Here's how the part is built. I have some questions about the finished solid (model axes, mm). Coordinates: 2 decimals unless noted, no trailing zeros. Write each loop counter-clockwise with the first axis right and the second up, starting at its lowest first coordinate (ties: lowest second). Pieces come first, ordered by that corner, then holes.
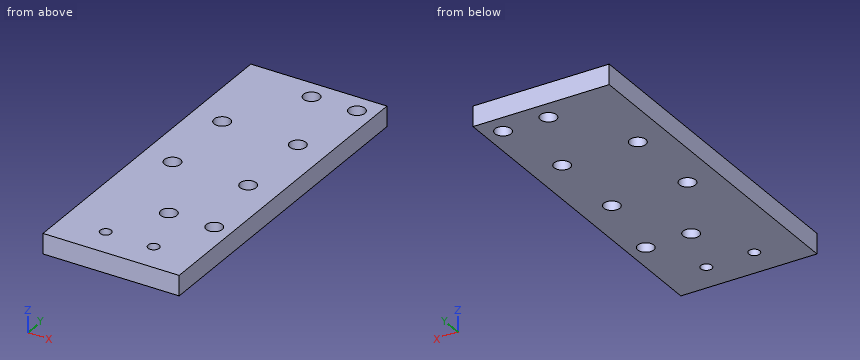
Autodesk Inventor part; units mm, degrees
ref_plane "YZ Plane" through (0, 0, 0) normal (1, 0, 0) x (0, 1, 0)
ref_plane "XZ Plane" through (0, 0, 0) normal (0, 1, 0) x (-1, 0, 0)
ref_plane "XY Plane" through (0, 0, 0) normal (0, 0, 1) x (1, 0, 0)
sketch "Эскиз1" plane through (0, 0, 0) normal (0, 0, 1) x (1, 0, 0)
  circle A0 centre (-7.5, -6.95) radius 1.5 construction
  circle A1 centre (7.5, -6.95) radius 1.5 construction
  circle A2 centre (7.5, -22.95) radius 1.5 construction
  circle A3 centre (-7.5, -22.95) radius 1.5 construction
  circle A4 centre (-7.5, -6.95) radius 1.6
  circle A5 centre (7.5, -6.95) radius 1.6
  circle A6 centre (7.5, -22.95) radius 1.6
  circle A7 centre (-7.5, -22.95) radius 1.6
  line L0 (9, 4.1) -> (-9, 4.1) construction
  line L1 (9, -34) -> (-9, -34) construction
  line L2 (-13.5, 12.05) -> (13.5, 12.05)
  line L3 (13.5, 12.05) -> (13.5, -41.95)
  line L4 (13.5, -41.95) -> (-13.5, -41.95)
  line L5 (-13.5, -41.95) -> (-13.5, 12.05)
  line L6 (-7.5, -6.95) -> (-7.5, 12.05) construction
  line L7 (-7.5, -22.95) -> (-7.5, -41.95) construction
  point P0 (0, 0)
  dimension "d0" = 3.2
  dimension "d1" = 3.2
  dimension "d2" = 3.2
  dimension "d3" = 3.2
  dimension "d4" = 6
  dimension "d5" = 6
  dimension "d8" = 54
extrude "Выдавливание1" add sketch "Эскиз1" along normal blind 4
sketch "Эскиз3" plane through (0, 0, 4) normal (0, 0, 1) x (1, 0, 0)
  circle A0 centre (1, -37.95) radius 2.1 construction
  circle A1 centre (10, -37.95) radius 2.1 construction
  circle A2 centre (1, 8.05) radius 2.1 construction
  circle A3 centre (10, 8.05) radius 2.1 construction
  circle A4 centre (1, -37.95) radius 1.6
  circle A5 centre (10, -37.95) radius 1.6
  circle A6 centre (1, 8.05) radius 1.6
  circle A7 centre (10, 8.05) radius 1.6
  point P0 (0, 0)
  dimension "d9" = 3.2
  dimension "d10" = 3.2
  dimension "d11" = 3.2
  dimension "d12" = 3.2
extrude "Выдавливание2" cut sketch "Эскиз3" against normal blind 10
sketch "Эскиз4" plane through (-13.5, -41.95, 0) normal (0, -1, 0) x (1, 0, 0)
  line L0 (0, 4) -> (27, 4)
  line L1 (0, 0) -> (0, 4)
  line L2 (0, 0) -> (27, 0)
  line L3 (27, 0) -> (27, 4)
  point P0 (13.5, 0)
extrude "Выдавливание3" add sketch "Эскиз4" along normal blind 13
sketch "Эскиз5" plane through (0, 0, 4) normal (0, 0, 1) x (1, 0, 0)
  circle A0 centre (-4.75, -48.95) radius 1.1
  circle A1 centre (4.75, -48.95) radius 1.1
  line L0 (13.5, -54.95) -> (-13.5, -54.95)
  line L1 (-4.75, -48.95) -> (4.75, -48.95) construction
  line L2 (-13.5, -54.95) -> (13.5, -54.95)
  line L3 (0, -54.95) -> (0, -44.9409) construction
  point P0 (0, 0)
  point P1 (0, -48.95)
  dimension "d17" = 2.2
  dimension "d18" = 2.2
  dimension "d19" = 6
  dimension "d20" = 6
  dimension "d21" = 9.5
extrude "Выдавливание4" cut sketch "Эскиз5" against normal blind 13
properties part number "фанера_каретка" material "Древесина (береза)"
1) I need wall thicknesses on probe 1 along Y at (x, z) = (10, 2.15); probe 2 along Y at (x, z) = (-7.5, 3.15); probe 3 along Y at (x, z) = (-4.75, 1.55). Which ranges of each line are inside material? Lowest first, please.
Values follow:
probe 1: y = -54.95 to -39.55, -36.35 to 6.45, 9.65 to 12.05
probe 2: y = -54.95 to -24.55, -21.35 to -8.55, -5.35 to 12.05
probe 3: y = -54.95 to -50.05, -47.85 to 12.05
2) Imagine slicing it at D-D on x = -4.75. Please give me the cut outline in (y, z), then the cut area to 3 significant figures.
Values follow:
outline: (-54.95, 0) - (-50.05, 0) - (-50.05, 4) - (-54.95, 4) - close; (-47.85, 0) - (12.05, 0) - (12.05, 4) - (-47.85, 4) - close
area: 259 mm2
3) Imagine slicing it at B-B on y = -22.95. Please give me the cut outline in (x, z), then the cut area to 3 significant figures.
Values follow:
outline: (-13.5, 0) - (-9.1, 0) - (-9.1, 4) - (-13.5, 4) - close; (-5.9, 0) - (5.9, 0) - (5.9, 4) - (-5.9, 4) - close; (9.1, 0) - (13.5, 0) - (13.5, 4) - (9.1, 4) - close
area: 82.4 mm2
4) Will this pin go through, and if not, where does the flat tip stop? pin 1 (2.5 mm diameter, centred on x = -7.5, y = -22.95, fed in from +Z).
Values follow:
pin 1: passes through
5) Imagine slicing it at A-A on x = 1. Please give me the cut outline in (y, z).
Values follow:
outline: (-54.95, 0) - (-39.55, 0) - (-39.55, 4) - (-54.95, 4) - close; (-36.35, 0) - (6.45, 0) - (6.45, 4) - (-36.35, 4) - close; (9.65, 0) - (12.05, 0) - (12.05, 4) - (9.65, 4) - close
6) Imagine slicing it at C-C on z = 1.1. Count the separate pieces of the cut face and the enclosed holes in it, then the cut area to 3 significant figures.
Values follow:
separate pieces: 1
enclosed holes: 10
area: 1,740 mm2
